Input: part model. Units: mm. Frame: model coordinates. Face numbers are marked on the shaded views. A direction names the side the tool comes from. Round coordinates to 2 decimals unless told otherwise and drop trailing zeros. Order: outer loops, then holes, each group sorted by start corner. A loop starts at its lowest first (then second) coordinate and runs counter-clockwise, first axis right, second up. Notation, with made-up numbers: M 62.5,3 L 103.5,3 A14 ccw 103.5,18 Z; hole C 60.5,-21 d6. An arc over 180 degrees is marked long. One line per question, with ' | ' between items.
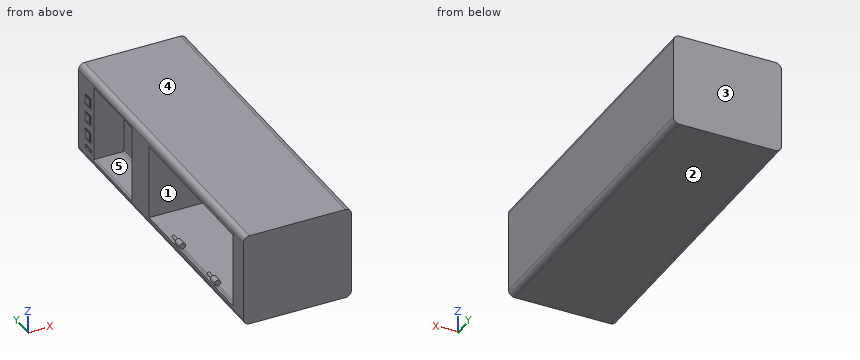
```python
from build123d import *

# Parameters (mm, degrees)
BOSS_EXTRUDE1_DEPTH  = 310
SKETCH2_W            = 250
SKETCH2_H            = 250
CUT_EXTRUDE3_DEPTH   = 100
SKETCH4_W            = 250
SKETCH4_H            = 550
CUT_EXTRUDE4_DEPTH   = 300
FILLET1_R            = 20
FILLET3_R            = 5
SKETCH6_W            = 34
SKETCH6_H            = 34
SKETCH6_W_2          = 30
SKETCH6_H_2          = 30
BOSS_EXTRUDE4_DEPTH  = 2
SKETCH8_W            = 26
SKETCH8_H            = 26
BOSS_EXTRUDE5_DEPTH  = 2
SKETCH9_R            = 2.5
BOSS_EXTRUDE6_DEPTH  = 2
SKETCH10_R           = 2.5
BOSS_EXTRUDE7_DEPTH  = 3
SKETCH17_R           = 10
BOSS_EXTRUDE15_DEPTH = 150
SKETCH19_R           = 10
CUT_EXTRUDE5_DEPTH   = 120
SKETCH20_R           = 5
BOSS_EXTRUDE16_DEPTH = 30
SKETCH22_R           = 10
BOSS_EXTRUDE20_DEPTH = 200
SKETCH27_R           = 10
CUT_EXTRUDE7_DEPTH   = 170
SKETCH28_R           = 5
BOSS_EXTRUDE21_DEPTH = 30


with BuildPart() as part:
    # Sketch1 → Boss-Extrude1 (new body)
    with BuildSketch(Plane.XY):
        Polygon((-360, -166.674176782), (-360, -422.512102988), (0, -422.512102988), (0, 657.487897012), (-360, 657.487897012), align=None)
    extrude(amount=BOSS_EXTRUDE1_DEPTH)

    # Sketch2 → Cut-Extrude3 (cut)
    with BuildSketch(Plane.ZY.offset(360)):
        with Locations((155, 432.487897012)):
            Rectangle(SKETCH2_W, SKETCH2_H)
    extrude(amount=-CUT_EXTRUDE3_DEPTH, mode=Mode.SUBTRACT)

    # Sketch4 → Cut-Extrude4 (cut)
    with BuildSketch(Plane.ZY.offset(360)):
        with Locations((155, -79.051121205)):
            Rectangle(SKETCH4_W, SKETCH4_H)
    extrude(amount=-CUT_EXTRUDE4_DEPTH, mode=Mode.SUBTRACT)

    # Fillet1
    fillet1_edges = [part.edges().sort_by_distance(p)[0] for p in [
        (0, 117.487897012, 310),
        (0, 117.487897012, 0),
        (-360, 117.487897012, 0),
        (-360, 117.487897012, 310),
    ]]
    fillet(fillet1_edges, radius=FILLET1_R)

    # Fillet3
    fillet3_edges = [part.edges().sort_by_distance(p)[0] for p in [
        (-260, 432.487897012, 30),
        (-260, 432.487897012, 280),
        (-360, 432.487897012, 30),
        (-360, 432.487897012, 280),
        (-60, -79.051121205, 30),
        (-60, -79.051121205, 280),
    ]]
    fillet(fillet3_edges, radius=FILLET3_R)

    # Sketch6 → Boss-Extrude4 (add)
    # profile 1 of 3: a face of its own
    with BuildSketch(Plane.ZY.offset(360)):
        with Locations((94.240330872, 593.82204287)):
            Rectangle(SKETCH6_W, SKETCH6_H)
        with Locations((94.240330872, 593.82204287)):
            Rectangle(SKETCH6_W_2, SKETCH6_H_2, mode=Mode.SUBTRACT)
    # profile 2 of 3: a face of its own
    with BuildSketch(Plane.ZY.offset(360)):
        with Locations((154.240330872, 593.82204287)):
            Rectangle(SKETCH6_W, SKETCH6_H)
        with Locations((154.240330872, 593.82204287)):
            Rectangle(SKETCH6_W_2, SKETCH6_H_2, mode=Mode.SUBTRACT)
    # profile 3 of 3: a face of its own
    with BuildSketch(Plane.ZY.offset(360)):
        with Locations((214.240330872, 593.82204287)):
            Rectangle(SKETCH6_W, SKETCH6_H)
        with Locations((214.240330872, 593.82204287)):
            Rectangle(SKETCH6_W_2, SKETCH6_H_2, mode=Mode.SUBTRACT)
    extrude(amount=BOSS_EXTRUDE4_DEPTH)

    # Sketch8 → Boss-Extrude5 (add)
    with BuildSketch(Plane.ZY.offset(360)):
        with Locations((94.240330872, 593.82204287)):
            Rectangle(SKETCH8_W, SKETCH8_H)
        with Locations((154.240330872, 593.82204287)):
            Rectangle(SKETCH8_W, SKETCH8_H)
        with Locations((214.240330872, 593.82204287)):
            Rectangle(SKETCH8_W, SKETCH8_H)
    extrude(amount=BOSS_EXTRUDE5_DEPTH)

    # Sketch9 → Boss-Extrude6 (add)
    with BuildSketch(Plane.ZY.offset(360)):
        with BuildLine():
            Line((42.525828736, 578.446941707), (42.525828736, 608.446941707))
            ThreePointArc((42.525828736, 608.446941707), (48.500463489, 614.42157646), (54.475098242, 608.446941707))
            Line((54.475098242, 608.446941707), (54.475098242, 578.446941707))
            ThreePointArc((54.475098242, 578.446941707), (48.500463489, 572.472306954), (42.525828736, 578.446941707))
        make_face()
        with Locations(Location((48.500463489, 604.166154606, 0), (0, 0, 270))):
            Circle(SKETCH9_R, mode=Mode.SUBTRACT)
        with Locations(Location((48.500463489, 583.02259952, 0), (0, 0, 270))):
            Circle(SKETCH9_R, mode=Mode.SUBTRACT)
    extrude(amount=BOSS_EXTRUDE6_DEPTH)

    # Sketch10 → Boss-Extrude7 (add)
    with BuildSketch(Plane.ZY.offset(360)):
        with Locations(Location((48.500463489, 604.166154606, 0), (0, 0, 270))):
            Circle(SKETCH10_R)
        with Locations(Location((48.500463489, 583.02259952, 0), (0, 0, 270))):
            Circle(SKETCH10_R)
    extrude(amount=BOSS_EXTRUDE7_DEPTH)

    # Sketch17 → Boss-Extrude15 (add)
    with BuildSketch(Plane(origin=(0, -354.051121205, 0), x_dir=(1, 0, 0), z_dir=(0, 1, 0))):
        with Locations((-349.825795865, -39.522123793)):
            Circle(SKETCH17_R)
    extrude(amount=BOSS_EXTRUDE15_DEPTH)

    # Sketch19 → Cut-Extrude5 (cut)
    with BuildSketch(Plane(origin=(0, -354.051121205, 0), x_dir=(1, 0, 0), z_dir=(0, 1, 0))):
        with Locations((-349.825795865, -39.522123793)):
            Circle(SKETCH19_R)
    extrude(amount=CUT_EXTRUDE5_DEPTH, mode=Mode.SUBTRACT)

    # Sketch20 → Boss-Extrude16 (add)
    with BuildSketch(Plane(origin=(0, -204.051121205, 0), x_dir=(1, 0, 0), z_dir=(0, 1, 0))):
        with Locations(Location((-349.825795865, -39.522123793, 0), (0, 0, 180))):
            Circle(SKETCH20_R)
    extrude(amount=BOSS_EXTRUDE16_DEPTH)

    # Sketch22 → Boss-Extrude20 (add)
    with BuildSketch(Plane(origin=(0, -174.051121205, 0), x_dir=(1, 0, 0), z_dir=(0, 1, 0))):
        with Locations((-349.825795865, -39.522123793)):
            Circle(SKETCH22_R)
    extrude(amount=BOSS_EXTRUDE20_DEPTH)

    # Sketch27 → Cut-Extrude7 (cut)
    with BuildSketch(Plane.XZ.offset(174.051121205)):
        with Locations((-349.825795865, 39.522123793)):
            Circle(SKETCH27_R)
    extrude(amount=-CUT_EXTRUDE7_DEPTH, mode=Mode.SUBTRACT)

    # Sketch28 → Boss-Extrude21 (add)
    with BuildSketch(Plane(origin=(0, 25.948878795, 0), x_dir=(1, 0, 0), z_dir=(0, 1, 0))):
        with Locations((-349.825795865, -39.522123793)):
            Circle(SKETCH28_R)
    extrude(amount=BOSS_EXTRUDE21_DEPTH)


solid = part.part
```
Item 1: Section query D-D, the plane x = -312.5. Return loops of the section in (y, z).
Report:
outline: M -422.51,0 L 657.49,0 L 657.49,310 L -422.51,310 Z; hole M -354.05,30 L 195.95,30 L 195.95,280 L -354.05,280 Z; hole M 307.49,30 L 557.49,30 L 557.49,280 L 307.49,280 Z
Item 2: Access query for the marked faces 1 and 2. Directions: +Z, -Z, +X, -X, +Y, -Y. A direction counts if a zero-diameter tool reaches every point of the face in a straight line with its end or side. Return the directions, or none.
Report:
face 1: -X | face 2: -Z, +X, -X, +Y, -Y
Item 3: Section query C-C, the plane y = -32. Return loops of the section in (x, z).
Report:
outline: M -360,20 A20 ccw -340,0 L -20,0 A20 ccw 0,20 L 0,290 A20 ccw -20,310 L -340,310 A20 ccw -360,290 L -360,280 L -65,280 A5 cw -60,275 L -60,35 A5 cw -65,30 L -346.77,30 A10 cw -352.88,30 L -360,30 Z
Item 4: Section query A-A, the plane x = -76. Return loops of the section in (y, z), plus the area to 3 significant figures.
Report:
outline: M -422.51,0 L 657.49,0 L 657.49,310 L -422.51,310 Z; hole M -354.05,30 L 195.95,30 L 195.95,280 L -354.05,280 Z | area: 197,000 mm²
Item 5: Line query: line 1 along Y through (x, z) = (-329, 49); line 2 along Z through (x, y) = (-316, -263.5); line 3 along Y through (x, z) = (-109.5, 105). Output: solid intervals per line, ascending. Write a range as from..to.
Report:
line 1: -422.51..-354.05, 195.95..307.49, 557.49..657.49 | line 2: 0..30, 280..310 | line 3: -422.51..-354.05, 195.95..657.49
Item 6: Mould query, pull axis Y, two halves, no side actions, for the marked faces 3, 4 and 5. Classes: +Y half, -Y half, draft (parallel to the pull), parting line (faces both ways), or undercut.
Report:
face 3: +Y half | face 4: draft | face 5: undercut
Item 7: Section query B-B, the plane z = 123.5. Return loops of the section in (x, y).
Report:
outline: M -360,-422.51 L 0,-422.51 L 0,657.49 L -360,657.49 L -360,557.49 L -260,557.49 L -260,307.49 L -360,307.49 L -360,195.95 L -60,195.95 L -60,-354.05 L -360,-354.05 Z
Item 8: First-contact query: pin 1 (1 mm diameter, centred on x = -361, y = 597.5, fed in from -Z); pin 2 (2 mm diameter, centred on x = -360.5, z = 97, fed in from +Y); pin 3 (6 mm diameter, centred on y = 200.5, z = 128.5, fed in from -X); pin 4 (1.6 mm diameter, centred on x = -361.5, z = 158, fed in from -Y). Flat tips, straight axial feed; report the tip coordinate or a pass-through.
Report:
pin 1: z = 42.53 | pin 2: y = 657.49 | pin 3: x = -360 | pin 4: y = 576.82
